Autodesk Inventor part; units mm, degrees
ref_plane "YZ Plane" through (0, 0, 0) normal (1, 0, 0) x (0, 1, 0)
ref_plane "XZ Plane" through (0, 0, 0) normal (0, 1, 0) x (-1, 0, 0)
ref_plane "XY Plane" through (0, 0, 0) normal (0, 0, 1) x (1, 0, 0)
sketch "スケッチ1" plane through (0, 0, 0) normal (0, 0, 1) x (1, 0, 0)
  line L0 (-10, 1.5) -> (10, 1.5)
  line L1 (10, 1.5) -> (10, -1.5)
  line L2 (10, -1.5) -> (-10, -1.5)
  line L3 (-10, -1.5) -> (-10, 1.5)
  line L4 (-10, 1.5) -> (10, -1.5) construction
  line L5 (10, 1.5) -> (-10, -1.5) construction
  point P0 (0, 0)
  dimension "d0" = 20
  dimension "d1" = 3
extrude "押し出し1" add sketch "スケッチ1" along normal blind 5
sketch "スケッチ2" plane through (-10, 1.5, 0) normal (0, 1, 0) x (1, 0, 0)
  line L0 (0, 0) -> (20, 0)
  line L1 (0, 0) -> (0, -5)
  line L2 (20, -5) -> (0, -5)
  line L3 (20, 0) -> (20, -5)
  line L4 (17, -2.5) -> (3, -2.5)
  line L5 (0, 0) -> (0, -5)
  point P0 (10, 0)
  point P1 (10, -5)
  point P2 (10, -2.5)
  point P3 (0, -2.5)
  dimension "d4" = 14
hole "穴1" at (-7, 1.5, 2.5) at (7, 1.5, 2.5) direction (0, -1, 0) diameter 2.459 depth 8.8 tip angle 118
properties part number "Key1"
For this review, take the finished solid that the model builds, in its own axes (mm). Round coordinates to 2 decimals unless told otherwise and drop trailing zeros. Order: outer loops, then holes, each group sorted by start corner. A loop starts at its lowest first (then second) coordinate and runs counter-clockwise, first axis right, second up. Notation, with made-up numbers: (49.25, -21) -> (85.25, -21) arc R19 cw to (85.25, -6) -> close; hole circle Ø5 at (-8, -28). An arc over 180 degrees is marked (long way). Write item = value, one per line. Start each with the question number.
1) The part is to be moulded in two halves that separate along Z. For faces 1 (the face through (0, 0, 0)), 2 (the face through (-5.91, -0.02, 3.07)), 3 (the face through (0, -1.5, 2)), say which applies: +Z half, -Z half, draft (parallel to the pull), parting line (faces both ways), or undercut.
2) To check wall thickness, follow line 1 (X direction, y = -1.35, z = 2.5); line 2 (Z direction, x = 7, y = 0.3); line 3 (Z direction, x = 8, y = -0.85). State the ranges of each line that lie inside material, in increasing order. Write a range as from..to.
3) Take a section at A-A on x = 7. State the section outline as (y, z) points.
4) Take a section at C-C on y = 0.75. State the section outline as (x, z) points, plus the area to 3 significant figures.
5) Take a section at D-D on z = 3.45. State the section outline as (x, y) points, plus the area to 3 significant figures.
6) Take a section at B-B on z = 2.5. State the section outline as (x, y) points.
Verdict:
q1.face_1 = -Z half
q1.face_2 = undercut
q1.face_3 = draft
q2.line_1 = -10..-8.23, -5.77..5.77, 8.23..10
q2.line_2 = 0..1.27, 3.73..5
q2.line_3 = 0..1.78, 3.22..5
q3.outline = (-1.5, 0) -> (1.5, 0) -> (1.5, 1.27) -> (-1.5, 1.27) -> close; (-1.5, 3.73) -> (1.5, 3.73) -> (1.5, 5) -> (-1.5, 5) -> close
q4.outline = (-10, 0) -> (10, 0) -> (10, 5) -> (-10, 5) -> close; hole circle Ø2.46 at (-7, 2.5); hole circle Ø2.46 at (7, 2.5)
q4.area = 90.5 mm2
q5.outline = (-10, -1.5) -> (-7.78, -1.5) -> (-7.78, 1.5) -> (-10, 1.5) -> close; (-6.22, -1.5) -> (6.22, -1.5) -> (6.22, 1.5) -> (-6.22, 1.5) -> close; (7.78, -1.5) -> (10, -1.5) -> (10, 1.5) -> (7.78, 1.5) -> close
q5.area = 50.6 mm2
q6.outline = (-10, -1.5) -> (-8.23, -1.5) -> (-8.23, 1.5) -> (-10, 1.5) -> close; (-5.77, -1.5) -> (5.77, -1.5) -> (5.77, 1.5) -> (-5.77, 1.5) -> close; (8.23, -1.5) -> (10, -1.5) -> (10, 1.5) -> (8.23, 1.5) -> close
